from build123d import *

# Parameters (mm, degrees)
SKETCH7_W           = 22
SKETCH7_H           = 22
BOSS_EXTRUDE2_DEPTH = 50
DRAFT2_ANGLE        = 20
SHELL2_T            = -4.8


with BuildPart() as part:
    # Sketch7 → Boss-Extrude2 (new body)
    with BuildSketch(Plane.XY):
        with Locations((11, 11)):
            Rectangle(SKETCH7_W, SKETCH7_H)
    extrude(amount=BOSS_EXTRUDE2_DEPTH)

    # Draft2
    draft2_faces = [part.faces().sort_by_distance(p)[0] for p in [
        (22, 11, 25),
        (11, 0, 25),
        (0, 11, 25),
        (11, 22, 25),
    ]]
    draft(draft2_faces, Plane.XY.offset(50), DRAFT2_ANGLE)

    # Shell2
    shell2_openings = [part.faces().sort_by_distance(p)[0] for p in [
        (11, 11, 50),
        (11, 11, 0),
    ]]
    offset(amount=SHELL2_T, openings=shell2_openings, kind=Kind.INTERSECTION)


solid = part.part
Work out the finished part from the listing and answer in its coordinate system (mm). A direction names the side the tool comes from. Give positions to 0.01 mm unless a question says otherwise; leave off trailing zeros. Write each loop counter-clockwise with the first axis right and the second up, starting at its lowest first coordinate (ties: lowest second). Pieces come first, ordered by that corner, then holes. Notation, with made-up numbers: M -21.5,8 L 15.5,8 A20 ccw 15.5,28 Z; hole C 32.5,-11.5 d5. An arc over 180 degrees is marked long. Answer as CSV lines item,"result".
Q1. A cutting plane is placed at A-A on z = 17.5. Write down the section's boundary in (x, y).
A:
outline,"M -11.83,-11.83 L 33.83,-11.83 L 33.83,33.83 L -11.83,33.83 Z; hole M -6.72,-6.72 L 28.72,-6.72 L 28.72,28.72 L -6.72,28.72 Z"
Q2. A cutting plane is placed at C-C on x = -8.5. Write down the section's boundary in (y, z), plus the area to 3 significant figures.
A:
outline,"M -18.2,0 L -13.09,0 L -8.5,12.61 L 30.5,12.61 L 35.09,0 L 40.2,0 L 30.5,26.65 L -8.5,26.65 Z"
area,"748 mm²"
Q3. The mould has two halves that part along Y. Classify faces 3 (the flat face through (10.59, 33.25, 19.09)), 4 (the flat face through (10.663, -6.141, 19.094)), 5 (the flat face through (33.25, 10.59, 19.09)): +Y half, -Y half, draft (parallel to the pull), parting line (faces both ways), or undercut.
A:
face 3,"+Y half"
face 4,"undercut"
face 5,"draft"
Q4. A tool of negligible diameter and unlimited length cuts with its end or side. For faces 1 (the flat face through (-11.25, 10.59, 19.09)), 2 (the flat face through (10.663, 28.141, 19.094)), from which of +Z, -Z, +X, -X, +Y, -Y can it reach the whole face along a straight path? Write none if from no direction.
A:
face 1,"+Z, -X, +Y, -Y"
face 2,"-Z"
Q5. A cutting plane is placed at B-B on y = 26.5. Write down the section's boundary in (x, z).
A:
outline,"M -18.2,0 L -13.09,0 L -4.5,23.6 L 26.5,23.6 L 35.09,0 L 40.2,0 L 26.5,37.64 L -4.5,37.64 Z"
Q6. Find the intervals of material crossed by probe 1 along Y at (x, z) = (20, 15.5); probe 2 along X at (y, z) = (18.5, 15); probe 3 along X at (y, z) = (12, 42), in increasing order. Write a range as [from, to].
A:
probe 1,"y = [-12.56, -7.45], [29.45, 34.56]"
probe 2,"x = [-12.74, -7.63], [29.63, 34.74]"
probe 3,"x = [-2.91, 2.2], [19.8, 24.91]"
Q7. A cutting plane is placed at D-D on z = 9.5. Write down the section's boundary in (x, y), plus the area to 3 significant figures.
A:
outline,"M -14.74,-14.74 L 36.74,-14.74 L 36.74,36.74 L -14.74,36.74 Z; hole M -9.63,-9.63 L 31.63,-9.63 L 31.63,31.63 L -9.63,31.63 Z"
area,"948 mm²"
Q8. Given P1, Ø4, axis at y = 16.5, z = 22, coming from the -X side; P2, Ø12, axis at y = 21, z = 17, coming from the -X side; P3, Ø1, axis at y = 0.5, z = 16, coming from the -X side, each flat-ended and moving along its own axis, determine where each tip first touches the part or whether it passes through.
A:
P1,"stops at x = -10.92"
P2,"stops at x = -14.19"
P3,"stops at x = -12.56"
